from build123d import *

# Parameters (mm, degrees)
SKETCH1_R           = 1
BOSS_EXTRUDE1_DEPTH = 3
CUT_EXTRUDE4_DEPTH  = 1.5


with BuildPart() as part:
    # Sketch1 → Boss-Extrude1 (new body)
    with BuildSketch(Plane.XY.offset(3)):
        Polygon((-38, -69.5), (38, -69.5), (40, -67.5), (40, 67.5), (38, 69.5), (-38, 69.5), (-40, 67.5), (-40, -67.5), align=None)
        with Locations(Location((35, 49.5, 0), (0, 0, 180))):
            Circle(SKETCH1_R, mode=Mode.SUBTRACT)
        with Locations(Location((-35, -63.5, 0), (0, 0, 180))):
            Circle(SKETCH1_R, mode=Mode.SUBTRACT)
        with Locations(Location((35, 63.5, 0), (0, 0, 180))):
            Circle(SKETCH1_R, mode=Mode.SUBTRACT)
        with Locations(Location((-35, -49.5, 0), (0, 0, 180))):
            Circle(SKETCH1_R, mode=Mode.SUBTRACT)
        with Locations(Location((-35, 49.5, 0), (0, 0, 180))):
            Circle(SKETCH1_R, mode=Mode.SUBTRACT)
        with Locations(Location((-35, 63.5, 0), (0, 0, 180))):
            Circle(SKETCH1_R, mode=Mode.SUBTRACT)
        with Locations(Location((35, -49.5, 0), (0, 0, 180))):
            Circle(SKETCH1_R, mode=Mode.SUBTRACT)
        with Locations(Location((35, -63.5, 0), (0, 0, 180))):
            Circle(SKETCH1_R, mode=Mode.SUBTRACT)
    extrude(amount=-BOSS_EXTRUDE1_DEPTH)

    # Sketch2 → Cut-Extrude4 (cut)
    with BuildSketch(Plane(origin=(0, 0, 0), x_dir=(-1, 0, 0), z_dir=(0, 0, -1))):
        with BuildLine():
            Line((1.706764898, 46.272292783), (1.706764898, 38.686671015))
            ThreePointArc((1.706764898, 38.686671015), (0, 36.979906118), (-1.706764898, 38.686671015))
            Line((-1.706764898, 38.686671015), (-1.706764898, 46.272292783))
            ThreePointArc((-1.706764898, 46.272292783), (0, 47.979057681), (1.706764898, 46.272292783))
        make_face()
        with BuildLine():
            Line((1.706764898, 3.792810884), (1.706764898, -3.792810884))
            ThreePointArc((1.706764898, -3.792810884), (0, -5.499575782), (-1.706764898, -3.792810884))
            Line((-1.706764898, -3.792810884), (-1.706764898, 3.792810884))
            ThreePointArc((-1.706764898, 3.792810884), (0, 5.499575782), (1.706764898, 3.792810884))
        make_face()
        with BuildLine():
            Line((-33.566376322, 46.272292783), (-33.566376322, 38.686671015))
            ThreePointArc((-33.566376322, 38.686671015), (-35.27314122, 36.979906118), (-36.979906118, 38.686671015))
            Line((-36.979906118, 38.686671015), (-36.979906118, 46.272292783))
            ThreePointArc((-36.979906118, 46.272292783), (-35.27314122, 47.979057681), (-33.566376322, 46.272292783))
        make_face()
        with BuildLine():
            Line((37.169546662, 46.272292783), (37.169546662, 38.686671015))
            ThreePointArc((37.169546662, 38.686671015), (35.462781764, 36.979906118), (33.756016866, 38.686671015))
            Line((33.756016866, 38.686671015), (33.756016866, 46.272292783))
            ThreePointArc((33.756016866, 46.272292783), (35.462781764, 47.979057681), (37.169546662, 46.272292783))
        make_face()
        with BuildLine():
            Line((1.706764898, -41.15199809), (1.706764898, -48.737619858))
            ThreePointArc((1.706764898, -48.737619858), (0, -50.444384755), (-1.706764898, -48.737619858))
            Line((-1.706764898, -48.737619858), (-1.706764898, -41.15199809))
            ThreePointArc((-1.706764898, -41.15199809), (0, -39.445233192), (1.706764898, -41.15199809))
        make_face()
        with BuildLine():
            Line((-33.566376322, -41.15199809), (-33.566376322, -48.737619858))
            ThreePointArc((-33.566376322, -48.737619858), (-35.27314122, -50.444384755), (-36.979906118, -48.737619858))
            Line((-36.979906118, -48.737619858), (-36.979906118, -41.15199809))
            ThreePointArc((-36.979906118, -41.15199809), (-35.27314122, -39.445233192), (-33.566376322, -41.15199809))
        make_face()
        with BuildLine():
            Line((-33.566376322, 3.792810884), (-33.566376322, -3.792810884))
            ThreePointArc((-33.566376322, -3.792810884), (-35.27314122, -5.499575782), (-36.979906118, -3.792810884))
            Line((-36.979906118, -3.792810884), (-36.979906118, 3.792810884))
            ThreePointArc((-36.979906118, 3.792810884), (-35.27314122, 5.499575782), (-33.566376322, 3.792810884))
        make_face()
        with BuildLine():
            Line((37.169546662, -41.15199809), (37.169546662, -48.737619858))
            ThreePointArc((37.169546662, -48.737619858), (35.462781764, -50.444384755), (33.756016866, -48.737619858))
            Line((33.756016866, -48.737619858), (33.756016866, -41.15199809))
            ThreePointArc((33.756016866, -41.15199809), (35.462781764, -39.445233192), (37.169546662, -41.15199809))
        make_face()
        with BuildLine():
            Line((37.169546662, 3.792810884), (37.169546662, -3.792810884))
            ThreePointArc((37.169546662, -3.792810884), (35.462781764, -5.499575782), (33.756016866, -3.792810884))
            Line((33.756016866, -3.792810884), (33.756016866, 3.792810884))
            ThreePointArc((33.756016866, 3.792810884), (35.462781764, 5.499575782), (37.169546662, 3.792810884))
        make_face()
    extrude(amount=-CUT_EXTRUDE4_DEPTH, mode=Mode.SUBTRACT)


solid = part.part
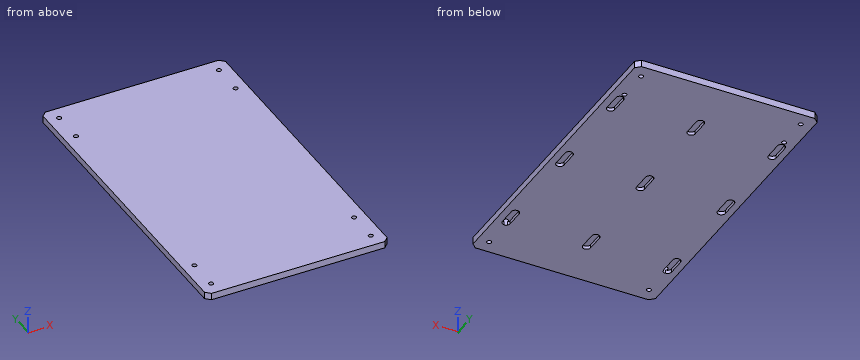
Read the model definition and answer for the solid it produces. Units are mm, in the model's axes. Round coordinates to 2 decimals unless told otherwise and drop trailing zeros. Loops run counter-clockwise (first coordinate to the right, second up) from the corner with the lowest first, then second, coordinate; pieces in that order, holes last.
Q1. Each of these flat-tipped pins is pushed along its axis until it touches: pin 1 (3 mm diameter, centred on x = -35, y = -63.5, fed in from -Z); pin 2 (1.6 mm diameter, centred on x = -35, y = -49.5, fed in from +Z). Where does it stop, or does it pass through?
Q2. Consider probe 1 along Y at (x, z) = (35, 1.7); probe 2 along Z at (x, y) = (36, -1). Determine where each line is inside the solid, lowest interval first.
Q3. Section A-A on x = 0 is taken. Write down the section's boundary in (y, z).
Output:
1. pin 1: stops at z = 0
1. pin 2: passes through
2. probe 1: y = -69.5 to -64.5, -62.5 to -50.5, -48.5 to 48.5, 50.5 to 62.5, 64.5 to 69.5
2. probe 2: z = 1.5 to 3
3. outline: (-69.5, 0) - (-50.44, 0) - (-50.44, 1.5) - (-39.45, 1.5) - (-39.45, 0) - (-5.5, 0) - (-5.5, 1.5) - (5.5, 1.5) - (5.5, 0) - (36.98, 0) - (36.98, 1.5) - (47.98, 1.5) - (47.98, 0) - (69.5, 0) - (69.5, 3) - (-69.5, 3) - close
